The listing builds one solid part. Answer for the finished solid, in the listing's coordinates (mm). A direction names the side the tool comes from. Round coordinates to 2 decimals unless told otherwise and drop trailing zeros. Loops run counter-clockwise (first coordinate to the right, second up) from the corner with the lowest first, then second, coordinate; pieces in that order, holes last. Notation, with made-up numbers: (2.25, -13.75) -> (8.25, -13.75) arc R15 ccw to (8.25, -6.75) -> close; hole circle Ø2 at (5, -40). An arc over 180 degrees is marked (long way). Answer in a Markdown table with one row per item. Add a question column.
```python
from build123d import *

# Parameters (mm, degrees)
SKETCH1_W            = 175
SKETCH1_H            = 55
BOSS_EXTRUDE1_DEPTH  = 10
SKETCH2_W            = 27.5
SKETCH2_H            = 55
BOSS_EXTRUDE2_DEPTH  = 10
M8_CLEARANCE_HOLE1_D = 10
M6_CLEARANCE_HOLE1_D = 7
FILLET1_R            = 10
SKETCH11_W           = 42.4
SKETCH11_H           = 42.4
CUT_EXTRUDE3_DEPTH   = 119.664442863
SKETCH12_R           = 4
CUT_EXTRUDE4_DEPTH   = 119.664442863
SKETCH13_W           = 5
SKETCH13_H           = 42.4
CUT_EXTRUDE5_DEPTH   = 119.664442863
CUT_EXTRUDE6_DEPTH   = 12.7
SKETCH16_R           = 2.7
CUT_EXTRUDE8_DEPTH   = 119.664442863


with BuildPart() as part:
    # Sketch1 → Boss-Extrude1 (new body)
    with BuildSketch(Plane(origin=(0, 0, 0), x_dir=(1, 0, 0), z_dir=(0, 1, 0))):
        Rectangle(SKETCH1_W, SKETCH1_H)
    extrude(amount=BOSS_EXTRUDE1_DEPTH)

    # Sketch2 → Boss-Extrude2 (add)
    with BuildSketch(Plane.XZ):
        with Locations((-101.25, 0)):
            Rectangle(SKETCH2_W, SKETCH2_H)
        with BuildLine():
            Line((87.5, 27.5), (87.5, -27.5))
            ThreePointArc((87.5, -27.5), (115, 0), (87.5, 27.5))
        make_face()
    extrude(amount=-BOSS_EXTRUDE2_DEPTH)

    # M8 Clearance Hole1 (through all)
    with Locations(Plane(origin=(0, 0, 0), x_dir=(-1, 0, 0), z_dir=(0, -1, 0))):
        with Locations((-87.5, 0)):
            Hole(M8_CLEARANCE_HOLE1_D / 2)

    # M6 Clearance Hole1 (through all)
    with Locations(Plane(origin=(0, 10, 0), x_dir=(1, 0, 0), z_dir=(0, 1, 0))):
        with Locations((87.5, 13), (74.5, 0), (100.5, 0), (87.5, -13)):
            Hole(M6_CLEARANCE_HOLE1_D / 2)

    # Fillet1
    fillet1_edges = [part.edges().sort_by_distance(p)[0] for p in [
        (-115, 5, -27.5),
        (-115, 5, 27.5),
    ]]
    fillet(fillet1_edges, radius=FILLET1_R)

    # Sketch11 → Cut-Extrude3 (cut, through all)
    with BuildSketch(Plane.XZ):
        with Locations((-3.7, 0)):
            Rectangle(SKETCH11_W, SKETCH11_H)
    extrude(amount=-CUT_EXTRUDE3_DEPTH, mode=Mode.SUBTRACT)

    # Sketch12 → Cut-Extrude4 (cut, through all)
    with BuildSketch(Plane.XZ):
        with Locations(Location((-78.9, 0, 0), (0, 0, 270))):
            Circle(SKETCH12_R)
    extrude(amount=-CUT_EXTRUDE4_DEPTH, mode=Mode.SUBTRACT)

    # Sketch13 → Cut-Extrude5 (cut, through all)
    with BuildSketch(Plane.XZ):
        Polygon((-25.1, -21.4), (-25.1, 21.4), (-24.9, 21.4), (-24.9, 21.2), (-24.9, -21.2), (-24.9, -21.4), align=None)
        Polygon((17.5, 21.2), (22.5, 21.2), (22.5, 21.4), (-24.9, 21.4), (-24.9, 21.2), align=None)
        with Locations((20, 0)):
            Rectangle(SKETCH13_W, SKETCH13_H)
        Polygon((-24.9, -21.2), (-24.9, -21.4), (22.5, -21.4), (22.5, -21.2), (17.5, -21.2), align=None)
    extrude(amount=-CUT_EXTRUDE5_DEPTH, mode=Mode.SUBTRACT)

    # Sketch14 → Cut-Extrude6 (cut)
    with BuildSketch(Plane.XZ):
        Polygon((91.541115254, 13.021371376), (100.521371376, 4.041115254), (105.011499436, 8.531243315), (96.031243315, 17.511499436), align=None)
    extrude(amount=-CUT_EXTRUDE6_DEPTH, mode=Mode.SUBTRACT)

    # Sketch16 → Cut-Extrude8 (cut, through all)
    with BuildSketch(Plane.XZ):
        with Locations(Location((-105, 17.5, 0), (0, 0, 270))):
            Circle(SKETCH16_R)
    extrude(amount=-CUT_EXTRUDE8_DEPTH, mode=Mode.SUBTRACT)


solid = part.part
```
Item 1: Flat-ended cylindrical pins translate along their axes: P1, Ø6, axis at y = 1.5, z = 16.5, coming from the +X side; P2, Ø1, axis at y = 9, z = -19.5, coming from the -X side. Find the tip coordinate at first contact, or state that the pin passes through.
Item 2: Section B-B, the plane z = 0 is taken. Write down the section's boundary in (x, y), and give its area (3 significant figures).
Item 3: Section C-C, the plane y = 4.25 is taken. Give the number of separate pieces and of enclosed holes in the cut face, and give its area (3 significant figures).
Item 4: The mould has two halves that part along X. Classify faces 3 (the cylindrical face through (71.267, 4.93, 1.341)), 4 (the cylindrical face through (114.993, 4.93, -0.605)), 5 (the flat face through (100.58, 4.93, 12.96)), 6 (the flat face through (-27, 0, 0)): +X half, -X half, draft (parallel to the pull), parting line (faces both ways), or undercut.
Item 5: Section D-D, the plane x = -7.5 is taken. Write down the section's boundary in (y, z), and give its area (3 significant figures).
Item 6: For faces 1 (the flat face through (-10, 5, 27.5)), 2 (the flat face through (-2, 5, -21.4)), determine the directions among +Z, -Z, +X, -X, +Y, -Y from which every point of the face is accessible in a straight line to the end or side of a thin tool.
Item 7: Section A-A, the plane x = 74.5 is taken. Write down the section's boundary in (y, z).
Item 8: Consider L1, parallel to Z at x = 87.5, y = 7; L2, parallel to X at y = 7, z = 0.5; L3, parallel to Z at x = -79, y = 3.5. Determine where each line is inside the solid, lowest interval first. Write a range as from..to.
Here are the results:
| question | item | result |
|---|---|---|
| 1 | P1 | stops at x = 111.46 |
| 1 | P2 | stops at x = -114.89 |
| 2 | outline | (-115, 0) -> (-82.9, 0) -> (-82.9, 10) -> (-115, 10) -> close; (-74.9, 0) -> (-25.1, 0) -> (-25.1, 10) -> (-74.9, 10) -> close; (22.5, 0) -> (71, 0) -> (71, 10) -> (22.5, 10) -> close; (78, 0) -> (82.5, 0) -> (82.5, 10) -> (78, 10) -> close; (92.5, 0) -> (97, 0) -> (97, 10) -> (92.5, 10) -> close; (104, 0) -> (115, 0) -> (115, 10) -> (104, 10) -> close |
| 2 | area | 1,500 mm² |
| 3 | separate pieces | 1 |
| 3 | enclosed holes | 9 |
| 3 | area | 9,860 mm² |
| 4 | face 3 | undercut |
| 4 | face 4 | +X half |
| 4 | face 5 | undercut |
| 4 | face 6 | draft |
| 5 | outline | (0, -27.5) -> (10, -27.5) -> (10, -21.4) -> (0, -21.4) -> close; (0, 21.4) -> (10, 21.4) -> (10, 27.5) -> (0, 27.5) -> close |
| 5 | area | 122 mm² |
| 6 | face 1 | +Z, +X, -X, +Y, -Y |
| 6 | face 2 | +Y, -Y |
| 7 | outline | (0, -27.5) -> (10, -27.5) -> (10, -3.5) -> (0, -3.5) -> close; (0, 3.5) -> (10, 3.5) -> (10, 27.5) -> (0, 27.5) -> close |
| 8 | L1 | z = -27.5..-16.5, -9.5..-5, 5..9.5, 16.5..27.5 |
| 8 | L2 | x = -115..-82.87, -74.93..-25.1, 22.5..71.04, 77.96..82.53, 92.47..97.04, 103.96..115 |
| 8 | L3 | z = -27.5..-4, 4..27.5 |
